Source: three-view drawing plus pictorial views. Frame: mm from the lowest corner of the part. A direction names the side the tool comes from. Give positions to 0.01 mm unless a question says otherwise; leave off trailing zeros. Loops run counter-clockwise (first coordinate to the right, second up) from the corner with the lowest first, then second, coordinate; pieces in that order, holes last.
1. First-contact query: P1, Ø2, axis at y = 7.5, z = 22, coming from the -X side. Flat tip, straight axial feed; report the tip coordinate or a pass-through.
2. Section A-A, the plane y = 6.75. Output: boundary loops of the cut face in (x, z), then the cut area to 3 significant figures.
3. Access query for the marked faces 1 and 2. Directions: +Z, -Z, +X, -X, +Y, -Y. A direction counts if a zero-diameter tool reaches every point of the face in a straight line with its end or side. Return the directions, or none.
4. Section C-C, the plane z = 11.5. Output: boundary loops of the cut face in (x, y), then the cut area to 3 significant figures.
5. Material intervals for line 1 along Z through (x, y) = (19.5, 5.75); line 2 along X through (y, z) = (7, 3.75), sorted ascending.
6. Section B-B, the plane x = 13.75. Output: boundary loops of the cut face in (y, z).
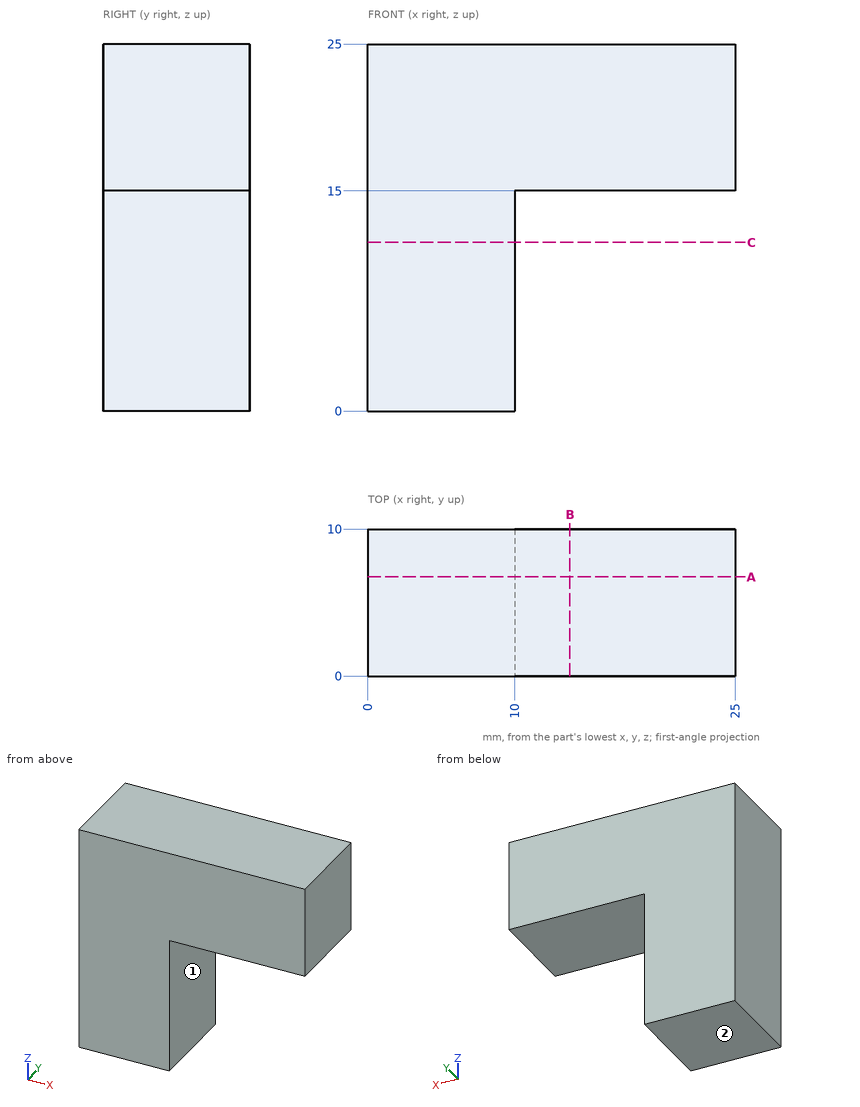
Answers below:
1. P1: stops at x = 0
2. outline: (0, 0) - (10, 0) - (10, 15) - (25, 15) - (25, 25) - (0, 25) - close
2. area: 400 mm2
3. face 1: -Z, +X, +Y, -Y
3. face 2: -Z, +X, -X, +Y, -Y
4. outline: (0, 0) - (10, 0) - (10, 10) - (0, 10) - close
4. area: 100 mm2
5. line 1: z = 15 to 25
5. line 2: x = 0 to 10
6. outline: (0, 15) - (10, 15) - (10, 25) - (0, 25) - close
